Here's how the part is built. I have some questions about the finished solid (model axes, mm). A direction names the side the tool comes from. Give positions to 0.01 mm unless a question says otherwise; leave off trailing zeros. Loops run counter-clockwise (first coordinate to the right, second up) from the corner with the lowest first, then second, coordinate; pieces in that order, holes last. Notation, with made-up numbers: (65.5, 78) - (124.5, 78) arc R15 ccw to (124.5, 94) - close; hole circle Ø5 at (-29.5, 4.5). An arc over 180 degrees is marked (long way). Use one line per item in the form item = value.
from build123d import *

# Parameters (mm, degrees)
BOSS_EXTRUDE1_DEPTH     = 3
FILLET1_R               = 2
SKETCH3_W               = 96
SKETCH3_H               = 152.5
BOSS_EXTRUDE2_DEPTH     = 3.9
CUT_EXTRUDE1_REACH      = 196.287
SKETCH4_R               = 1.75
CHAMFER1_SIZE           = 4
SKETCH5_R               = 5
SKETCH5_R_2             = 9
CUT_EXTRUDE2_DEPTH      = 195.204042265
FILLET2_R               = 1.5
SKETCH7_W               = 20
SKETCH7_H               = 20
SKETCH7_W_2             = 18
SKETCH7_H_2             = 18
BOSS_EXTRUDE3_DEPTH     = 3.9
CUT_EXTRUDE3_DEPTH      = 195.204042265
CROQUIS1_R              = 3
CROQUIS1_R_2            = 1.25
SALIENTE_EXTRUIR1_DEPTH = 5
CROQUIS2_R              = 3
CROQUIS2_R_2            = 1.25
CROQUIS2_W              = 22
CROQUIS2_H              = 3
SALIENTE_EXTRUIR2_DEPTH = 5.5
CORTAR_EXTRUIR1_REACH   = 196.243
CROQUIS3_R              = 26.5
CORTAR_EXTRUIR2_REACH   = 196.243
CROQUIS4_R              = 2.5
CROQUIS5_W              = 59
CROQUIS5_H              = 40
CORTAR_EXTRUIR3_DEPTH   = 2
CROQUIS6_W              = 58
CROQUIS6_H              = 31
CORTAR_EXTRUIR4_DEPTH   = 2


with BuildPart() as part:
    # Sketch1 → Boss-Extrude1 (new body)
    with BuildSketch(Plane.XY):
        with BuildLine():
            Line((0, 0), (110, 0))
            Line((110, 0), (110, 153))
            ThreePointArc((110, 153), (107.949747468, 157.949747468), (103, 160))
            Line((103, 160), (7, 160))
            ThreePointArc((7, 160), (2.050252532, 157.949747468), (0, 153))
            Line((0, 153), (0, 0))
        make_face()
    extrude(amount=BOSS_EXTRUDE1_DEPTH)

    # Fillet1
    fillet1_edges = [part.edges().sort_by_distance(p)[0] for p in [
        (110, 76.5, 3),
        (107.949747468, 157.949747468, 3),
        (55, 160, 3),
        (2.050252532, 157.949747468, 3),
        (0, 76.5, 3),
        (55, 0, 3),
    ]]
    fillet(fillet1_edges, radius=FILLET1_R)

    # Sketch3 → Boss-Extrude2 (add)
    with BuildSketch(Plane(origin=(0, 0, 0), x_dir=(-1, 0, 0), z_dir=(0, 0, -1))):
        with Locations((-55, 76.25)):
            Rectangle(SKETCH3_W, SKETCH3_H)
        with BuildLine():
            Line((-101.4, 1.6), (-101.4, 33.5))
            Line((-101.4, 33.5), (-97, 33.5))
            ThreePointArc((-97, 33.5), (-93, 37.5), (-97, 41.5))
            Line((-97, 41.5), (-101.4, 41.5))
            Line((-101.4, 41.5), (-101.4, 123.5))
            Line((-101.4, 123.5), (-97, 123.5))
            ThreePointArc((-97, 123.5), (-93, 127.5), (-97, 131.5))
            Line((-97, 131.5), (-101.4, 131.5))
            Line((-101.4, 131.5), (-101.4, 150.9))
            Line((-101.4, 150.9), (-8.6, 150.9))
            Line((-8.6, 150.9), (-8.6, 131.5))
            Line((-8.6, 131.5), (-13, 131.5))
            ThreePointArc((-13, 131.5), (-17, 127.5), (-13, 123.5))
            Line((-13, 123.5), (-8.6, 123.5))
            Line((-8.6, 123.5), (-8.6, 41.5))
            Line((-8.6, 41.5), (-13, 41.5))
            ThreePointArc((-13, 41.5), (-17, 37.5), (-13, 33.5))
            Line((-13, 33.5), (-8.6, 33.5))
            Line((-8.6, 33.5), (-8.6, 1.6))
            Line((-8.6, 1.6), (-101.4, 1.6))
        make_face(mode=Mode.SUBTRACT)
    extrude(amount=BOSS_EXTRUDE2_DEPTH)

    # Sketch4 → Cut-Extrude1 (cut, up to next)
    with BuildSketch(Plane(origin=(0, 0, -3.9), x_dir=(-1, 0, 0), z_dir=(0, 0, -1)), mode=Mode.PRIVATE) as cut_extrude1_sk1:
        with Locations((-97, 127.5)):
            Circle(SKETCH4_R)
    cut_extrude1_tool1 = extrude(cut_extrude1_sk1.sketch, amount=-CUT_EXTRUDE1_REACH, mode=Mode.PRIVATE) & part.part
    # Sketch4 → Cut-Extrude1 (cut, up to next)
    with BuildSketch(Plane(origin=(0, 0, -3.9), x_dir=(-1, 0, 0), z_dir=(0, 0, -1)), mode=Mode.PRIVATE) as cut_extrude1_sk2:
        with Locations((-13, 127.5)):
            Circle(SKETCH4_R)
    cut_extrude1_tool2 = extrude(cut_extrude1_sk2.sketch, amount=-CUT_EXTRUDE1_REACH, mode=Mode.PRIVATE) & part.part
    # Sketch4 → Cut-Extrude1 (cut, up to next)
    with BuildSketch(Plane(origin=(0, 0, -3.9), x_dir=(-1, 0, 0), z_dir=(0, 0, -1)), mode=Mode.PRIVATE) as cut_extrude1_sk3:
        with Locations((-13, 37.5)):
            Circle(SKETCH4_R)
    cut_extrude1_tool3 = extrude(cut_extrude1_sk3.sketch, amount=-CUT_EXTRUDE1_REACH, mode=Mode.PRIVATE) & part.part
    # Sketch4 → Cut-Extrude1 (cut, up to next)
    with BuildSketch(Plane(origin=(0, 0, -3.9), x_dir=(-1, 0, 0), z_dir=(0, 0, -1)), mode=Mode.PRIVATE) as cut_extrude1_sk4:
        with Locations((-97, 37.5)):
            Circle(SKETCH4_R)
    cut_extrude1_tool4 = extrude(cut_extrude1_sk4.sketch, amount=-CUT_EXTRUDE1_REACH, mode=Mode.PRIVATE) & part.part
    add(cut_extrude1_tool1.solids().sort_by_distance((97, 127.5, -3.9))[0], mode=Mode.SUBTRACT)
    add(cut_extrude1_tool2.solids().sort_by_distance((13, 127.5, -3.9))[0], mode=Mode.SUBTRACT)
    add(cut_extrude1_tool3.solids().sort_by_distance((13, 37.5, -3.9))[0], mode=Mode.SUBTRACT)
    add(cut_extrude1_tool4.solids().sort_by_distance((97, 37.5, -3.9))[0], mode=Mode.SUBTRACT)

    # Chamfer1
    chamfer1_edges = [part.edges().sort_by_distance(p)[0] for p in [
        (98.75, 37.5, 3),
        (14.75, 37.5, 3),
        (14.75, 127.5, 3),
        (98.75, 127.5, 3),
    ]]
    chamfer(chamfer1_edges, length=CHAMFER1_SIZE)

    # Sketch5 → Cut-Extrude2 (cut, through all)
    with BuildSketch(Plane(origin=(0, 0, 0), x_dir=(-1, 0, 0), z_dir=(0, 0, -1))):
        with Locations((-28.6, 137.9)):
            Circle(SKETCH5_R)
        with Locations((-81.4, 137.9)):
            Circle(SKETCH5_R_2)
    extrude(amount=-CUT_EXTRUDE2_DEPTH, mode=Mode.SUBTRACT)

    # Fillet2
    fillet2_edges = [part.edges().sort_by_distance(p)[0] for p in [
        (90.4, 137.9, 0),
    ]]
    fillet(fillet2_edges, radius=FILLET2_R)

    # Sketch7 → Boss-Extrude3 (add)
    with BuildSketch(Plane(origin=(0, 0, 0), x_dir=(-1, 0, 0), z_dir=(0, 0, -1))):
        with Locations((-55, 137.9)):
            Rectangle(SKETCH7_W, SKETCH7_H)
        with Locations((-55, 137.9)):
            Rectangle(SKETCH7_W_2, SKETCH7_H_2, mode=Mode.SUBTRACT)
    extrude(amount=BOSS_EXTRUDE3_DEPTH)

    # Sketch8 → Cut-Extrude3 (cut, through all)
    with BuildSketch(Plane(origin=(0, 0, 0), x_dir=(-1, 0, 0), z_dir=(0, 0, -1))):
        with BuildLine():
            Line((-62, 146.4), (-48, 146.4))
            ThreePointArc((-48, 146.4), (-47, 145.4), (-48, 144.4))
            Line((-48, 144.4), (-62, 144.4))
            ThreePointArc((-62, 144.4), (-63, 145.4), (-62, 146.4))
        make_face()
        with BuildLine():
            Line((-62, 142.8), (-48, 142.8))
            ThreePointArc((-48, 142.8), (-47, 141.8), (-48, 140.8))
            Line((-48, 140.8), (-62, 140.8))
            ThreePointArc((-62, 140.8), (-63, 141.8), (-62, 142.8))
        make_face()
        with BuildLine():
            Line((-62, 139.2), (-48, 139.2))
            ThreePointArc((-48, 139.2), (-47, 138.2), (-48, 137.2))
            Line((-48, 137.2), (-62, 137.2))
            ThreePointArc((-62, 137.2), (-63, 138.2), (-62, 139.2))
        make_face()
        with BuildLine():
            Line((-62, 135.6), (-48, 135.6))
            ThreePointArc((-48, 135.6), (-47, 134.6), (-48, 133.6))
            Line((-48, 133.6), (-62, 133.6))
            ThreePointArc((-62, 133.6), (-63, 134.6), (-62, 135.6))
        make_face()
        with BuildLine():
            Line((-62, 132), (-48, 132))
            ThreePointArc((-48, 132), (-47, 131), (-48, 130))
            Line((-48, 130), (-62, 130))
            ThreePointArc((-62, 130), (-63, 131), (-62, 132))
        make_face()
    extrude(amount=-CUT_EXTRUDE3_DEPTH, mode=Mode.SUBTRACT)

    # Croquis1 → Saliente-Extruir1 (add)
    with BuildSketch(Plane(origin=(0, 0, 0), x_dir=(-1, 0, 0), z_dir=(0, 0, -1))):
        with Locations((-28.6, 116.15)):
            Circle(CROQUIS1_R)
        with Locations((-28.6, 116.15)):
            Circle(CROQUIS1_R_2, mode=Mode.SUBTRACT)
    extrude(amount=SALIENTE_EXTRUIR1_DEPTH)

    # Croquis2 → Saliente-Extruir2 (add)
    # profile 1 of 3: a face of its own
    with BuildSketch(Plane(origin=(0, 0, 0), x_dir=(-1, 0, 0), z_dir=(0, 0, -1))):
        with Locations((-88.9, 120.4)):
            Circle(CROQUIS2_R)
        with Locations((-88.9, 120.4)):
            Circle(CROQUIS2_R_2, mode=Mode.SUBTRACT)
    # profile 2 of 3: a face of its own
    with BuildSketch(Plane(origin=(0, 0, 0), x_dir=(-1, 0, 0), z_dir=(0, 0, -1))):
        with Locations((-73.9, 120.4)):
            Circle(CROQUIS2_R)
        with Locations((-73.9, 120.4)):
            Circle(CROQUIS2_R_2, mode=Mode.SUBTRACT)
    # profile 3 of 3: a face of its own
    with BuildSketch(Plane(origin=(0, 0, 0), x_dir=(-1, 0, 0), z_dir=(0, 0, -1))):
        with Locations((-81.4, 149.4)):
            Rectangle(CROQUIS2_W, CROQUIS2_H)
    extrude(amount=SALIENTE_EXTRUIR2_DEPTH)

    # Croquis3 → Cortar-Extruir1 (cut, up to next)
    with BuildSketch(Plane(origin=(0, 0, 0), x_dir=(-1, 0, 0), z_dir=(0, 0, -1)), mode=Mode.PRIVATE) as cortar_extruir1_sk1:
        with Locations((-55.631510191, 41.6)):
            Circle(CROQUIS3_R)
    cortar_extruir1_tool1 = extrude(cortar_extruir1_sk1.sketch, amount=-CORTAR_EXTRUIR1_REACH, mode=Mode.PRIVATE) & part.part
    add(cortar_extruir1_tool1.solids().sort_by_distance((55.63151, 41.6, 0))[0], mode=Mode.SUBTRACT)

    # Croquis4 → Cortar-Extruir2 (cut, up to next)
    with BuildSketch(Plane(origin=(0, 0, 0), x_dir=(-1, 0, 0), z_dir=(0, 0, -1)), mode=Mode.PRIVATE) as cortar_extruir2_sk1:
        with Locations((-83.181762723, 69.150252532)):
            Circle(CROQUIS4_R)
    cortar_extruir2_tool1 = extrude(cortar_extruir2_sk1.sketch, amount=-CORTAR_EXTRUIR2_REACH, mode=Mode.PRIVATE) & part.part
    # Croquis4 → Cortar-Extruir2 (cut, up to next)
    with BuildSketch(Plane(origin=(0, 0, 0), x_dir=(-1, 0, 0), z_dir=(0, 0, -1)), mode=Mode.PRIVATE) as cortar_extruir2_sk2:
        with Locations((-28.081257659, 69.150252532)):
            Circle(CROQUIS4_R)
    cortar_extruir2_tool2 = extrude(cortar_extruir2_sk2.sketch, amount=-CORTAR_EXTRUIR2_REACH, mode=Mode.PRIVATE) & part.part
    # Croquis4 → Cortar-Extruir2 (cut, up to next)
    with BuildSketch(Plane(origin=(0, 0, 0), x_dir=(-1, 0, 0), z_dir=(0, 0, -1)), mode=Mode.PRIVATE) as cortar_extruir2_sk3:
        with Locations((-28.081257659, 14.049747468)):
            Circle(CROQUIS4_R)
    cortar_extruir2_tool3 = extrude(cortar_extruir2_sk3.sketch, amount=-CORTAR_EXTRUIR2_REACH, mode=Mode.PRIVATE) & part.part
    # Croquis4 → Cortar-Extruir2 (cut, up to next)
    with BuildSketch(Plane(origin=(0, 0, 0), x_dir=(-1, 0, 0), z_dir=(0, 0, -1)), mode=Mode.PRIVATE) as cortar_extruir2_sk4:
        with Locations((-83.181762723, 14.049747468)):
            Circle(CROQUIS4_R)
    cortar_extruir2_tool4 = extrude(cortar_extruir2_sk4.sketch, amount=-CORTAR_EXTRUIR2_REACH, mode=Mode.PRIVATE) & part.part
    add(cortar_extruir2_tool1.solids().sort_by_distance((83.181763, 69.150253, 0))[0], mode=Mode.SUBTRACT)
    add(cortar_extruir2_tool2.solids().sort_by_distance((28.081258, 69.150253, 0))[0], mode=Mode.SUBTRACT)
    add(cortar_extruir2_tool3.solids().sort_by_distance((28.081258, 14.049747, 0))[0], mode=Mode.SUBTRACT)
    add(cortar_extruir2_tool4.solids().sort_by_distance((83.181763, 14.049747, 0))[0], mode=Mode.SUBTRACT)

    # Croquis5 → Cortar-Extruir3 (cut)
    with BuildSketch(Plane(origin=(0, 0, 0), x_dir=(-1, 0, 0), z_dir=(0, 0, -1))):
        with Locations((-55, 95.542989332)):
            Rectangle(CROQUIS5_W, CROQUIS5_H)
    extrude(amount=-CORTAR_EXTRUIR3_DEPTH, mode=Mode.SUBTRACT)

    # Croquis6 → Cortar-Extruir4 (cut)
    with BuildSketch(Plane(origin=(0, 0, 2), x_dir=(-1, 0, 0), z_dir=(0, 0, -1))):
        with Locations((-55, 99.042989332)):
            Rectangle(CROQUIS6_W, CROQUIS6_H)
    extrude(amount=-CORTAR_EXTRUIR4_DEPTH, mode=Mode.SUBTRACT)


solid = part.part
(1) If we section it at B-B (z = -2.5): Give the number of separate pieces and of enclosed holes in the cut face, plus the area to 3 significant figures.
Geometry says:
separate_pieces = 5
enclosed_holes = 9
area = 1,200 mm²
(2) For P1, Ø0.8, axis at x = 89, y = 120.5, coming from the -Z side; P2, Ø4.5, axis at x = 13, y = 127.5, coming from the -Z side; P3, Ø5.5, axis at x = 97, y = 127.5, coming from the +Z side, each with a flat end and sliding along its axis, tell me the tip position at first contact or that it passes through.
Geometry says:
P1 = 0
P2 = -3.9
P3 = 0
(3) If we section it at D-D (y = 48): List the corners of the cut face in (x, z) for me, plus the area to 3 significant figures.
Geometry says:
outline = (0, 0) - (7, 0) - (7, -3.9) - (8.6, -3.9) - (8.6, 0) - (29.92, 0) - (29.92, 3) - (2, 3) arc R2 ccw to (0, 1) - close; (81.35, 0) - (101.4, 0) - (101.4, -3.9) - (103, -3.9) - (103, 0) - (110, 0) - (110, 1) arc R2 ccw to (108, 3) - (81.35, 3) - close
area = 186 mm²
(4) If we section it at C-C (x = 21.5): List the corners of the cut face in (y, z) for me.
Geometry says:
outline = (0, -3.9) - (1.6, -3.9) - (1.6, 0) - (150.9, 0) - (150.9, -3.9) - (152.5, -3.9) - (152.5, 0) - (160, 0) - (160, 1) arc R2 ccw to (158, 3) - (2, 3) arc R2 ccw to (0, 1) - close
(5) If we section it at A-A (x = 67): List the corners of the cut face in (y, z) for me, plus the area to 3 significant figures.
Geometry says:
outline = (0, -3.9) - (1.6, -3.9) - (1.6, 0) - (17.66, 0) - (17.66, 3) - (2, 3) arc R2 ccw to (0, 1) - close; (65.54, 0) - (75.54, 0) - (75.54, 2) - (83.54, 2) - (83.54, 3) - (65.54, 3) - close; (114.54, 2) - (115.54, 2) - (115.54, 0) - (150.9, 0) - (150.9, -3.9) - (152.5, -3.9) - (152.5, 0) - (160, 0) - (160, 1) arc R2 ccw to (158, 3) - (114.54, 3) - close
area = 236 mm²
(6) If I drill on probe 1 along Y at (x, z) = (13, -2.5); probe 2 along Y at (x, z) = (35, -3.25); probe 3 along X at (y, z) = (46.5, -1.25), over which ranges is the centre line in solid material (lowest first)?
Geometry says:
probe_1 = 0 to 1.6, 33.5 to 35.75, 39.25 to 41.5, 123.5 to 125.75, 129.25 to 131.5, 150.9 to 152.5
probe_2 = 0 to 1.6, 150.9 to 152.5
probe_3 = 7 to 8.6, 101.4 to 103
(7) Thinking about a two-plate mould opening in Y: for faces 1 (the flat face through (82, 149, -5.5)), 2 (the flat face through (56, 152.5, -2)), 3 (the flat face through (8.6, 141, -2)), which applies, pulls with the +Y half, pulls with the -Y half, needs draft (parallel to the pull), parting line crosses it, or undercut?
Geometry says:
face_1 = needs draft
face_2 = pulls with the +Y half
face_3 = undercut
(8) For faces 4 (the flat face through (74, 119, -5.5)), 5 (the flat face through (40, 150.9, -2)), 6 (the flat face through (55, 144.4, 1)), which set-ups out of +Z, -Z, +X, -X, +Y, -Y let a thin tool reach every point of the face, with its end or its side?
Geometry says:
face_4 = -Z, +X, -X, +Y, -Y
face_5 = -Z
face_6 = +Z, -Z
